Here's how the part is built. I have some questions about the finished solid (model axes, mm). Face numbers are marked on the shaded views. Coordinates: 2 decimals unless noted, no trailing zeros. Write each loop counter-clockwise with the first axis right and the second up, starting at its lowest first coordinate (ties: lowest second). Pieces come first, ordered by that corner, then holes.
Item 1: We'd pull the mould along Z, two halves only. Please class the marked faces 1, 2, 3 and 4: +Z half, -Z half, draft (parallel to the pull), parting line (faces both ways), or undercut.
Item 2: If we section it at B-B (z = 28): Please give me the cut outline in (x, y), then the cut area to 3 significant figures.
Item 3: If I drill on line 1 (X direction, y = 14, z = 31); line 2 (X direction, y = 11, z = 17); line 3 (Y direction, x = 97, z = 23.5), over which ranges is the centre line in solid material (lowest first)?
Item 4: If we section it at A-A (x = 90): Please give me the cut outline in (y, z), then the cut area to 3 significant figures.
Item 5: If we section it at C-C (y = 16): Please give me the cut outline in (x, z).
Autodesk Inventor part; units mm, degrees
ref_plane "YZ Plane" through (0, 0, 0) normal (1, 0, 0) x (0, 1, 0)
ref_plane "XZ Plane" through (0, 0, 0) normal (0, 1, 0) x (-1, 0, 0)
ref_plane "XY Plane" through (0, 0, 0) normal (0, 0, 1) x (1, 0, 0)
sketch "Sketch1" plane through (0, 0, 0) normal (0, 0, 1) x (1, 0, 0)
  line L0 (63.5852, 104.9902) -> (114.3852, 104.9902)
  line L1 (114.3852, 104.9902) -> (114.3852, 3.3902)
  line L2 (114.3852, 3.3902) -> (63.5852, 3.3902)
  line L3 (63.5852, 3.3902) -> (63.5852, 104.9902)
  point P0 (0, 0)
  dimension "d0" = 50.8
  dimension "d1" = 101.6
extrude "Extrusion1" add sketch "Sketch1" along normal blind 50.8
sketch "Sketch2" plane through (63.5852, 3.3902, 0) normal (0, -1, 0) x (1, 0, 0)
  circle A0 centre (25.8879, 25.992) radius 12.2628
  point P0 (-63.5852, 0)
extrude "Extrusion2" cut sketch "Sketch2" against normal blind 25.4
properties part number "laser" material "Iron, Cast"
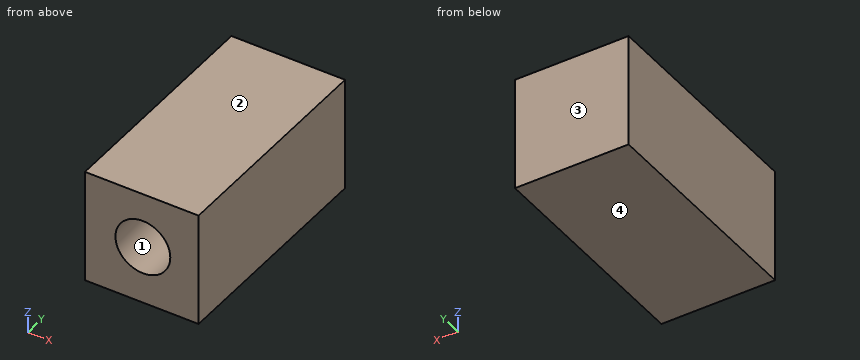
Answer list:
1. face 1: undercut
1. face 2: +Z half
1. face 3: draft
1. face 4: -Z half
2. outline: (63.59, 3.39) - (77.38, 3.39) - (77.38, 28.79) - (101.57, 28.79) - (101.57, 3.39) - (114.39, 3.39) - (114.39, 104.99) - (63.59, 104.99) - close
2. area: 4,550 mm2
3. line 1: x = 63.59 to 78.28, 100.67 to 114.39
3. line 2: x = 63.59 to 81.14, 97.81 to 114.39
3. line 3: y = 28.79 to 104.99
4. outline: (3.39, 0) - (104.99, 0) - (104.99, 50.8) - (3.39, 50.8) - (3.39, 38.24) - (28.79, 38.24) - (28.79, 13.74) - (3.39, 13.74) - close
4. area: 4,540 mm2
5. outline: (63.59, 0) - (114.39, 0) - (114.39, 50.8) - (63.59, 50.8) - close; hole circle Ø24.53 at (89.47, 25.99)
